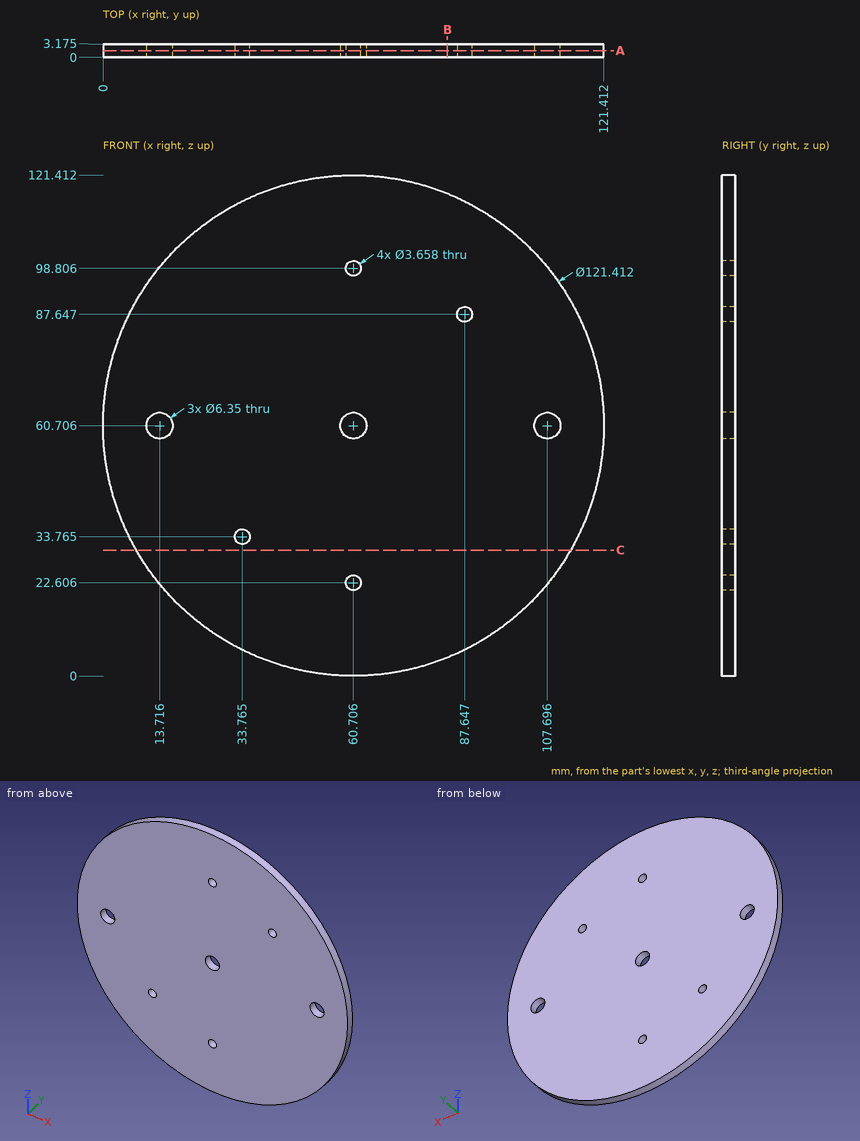
Design review of the part shown in the three views and the two pictorial views. Dimensions are in mm from the part's minimum x, y and z. Round coordinates to 2 decimals unless told otherwise and drop trailing zeros. Order: outer loops, then holes, each group sorted by start corner. A loop starts at its lowest first (then second) coordinate and runs counter-clockwise, first axis right, second up. Notation, with made-up numbers: (23.25, 62.25) - (39.25, 62.25) arc R23 cw to (39.25, 88.25) - close; hole circle Ø8 at (82, 71.5). An arc over 180 degrees is marked (long way). Answer in a Markdown table with one row per item.
(1) Take a section at B-B on x = 83.5. Write out the cut boundary in (y, z) (1 decimal).
Result set:
| item | result |
|---|---|
| outline | (0, 4.4) - (3.2, 4.4) - (3.2, 117) - (0, 117) - close |
(2) For line 1 (Z direction, x = 33, y = 1.2) (1 decimal); line 2 (Z direction, x = 110, y = 2.5) (1 decimal); line 3 (X direction, y = 1.85, z = 20), list the stretches that pass through material, from the lowest coordinate up. Write a range as from..to.
Result set:
| item | result |
|---|---|
| line 1 | z = 6.7..32.1, 35.4..114.7 |
| line 2 | z = 25.3..58.5, 62.9..96.1 |
| line 3 | x = 15.67..105.74 |
(3) Take a section at C-C on z = 30.5. Write out the cut boundary in (x, y) (1 decimal).
Result set:
| item | result |
|---|---|
| outline | (8, 0) - (113.4, 0) - (113.4, 3.2) - (8, 3.2) - close |
(4) Take a section at A-A on y = 1.55. Count the separate pieces of the cut face and the enclosed holes in it, plus the area to 3 significant figures.
Result set:
| item | result |
|---|---|
| separate pieces | 1 |
| enclosed holes | 7 |
| area | 11,400 mm2 |
(5) Clearance check with a flat-ended pin moving along its axis: P1, Ø1.5, axis at x = 80, y = 3, coming from the +Z side. State where the tip first meets the part, or that it passes through.
Result set:
| item | result |
|---|---|
| P1 | stops at z = 118.51 |
